Read the model definition and answer for the solid it produces. Units are mm, in the model's axes. Face numbers are marked on the shaded views. A direction names the side the tool comes from. Coordinates: 2 decimals unless noted, no trailing zeros. Order: outer loops, then holes, each group sorted by start corner. A loop starts at its lowest first (then second) coordinate and runs counter-clockwise, first axis right, second up. Notation, with made-up numbers: M 79.25,-24.75 L 115.25,-24.75 A25 ccw 115.25,11.25 Z; hole C -18.75,82.5 d5. An arc over 180 degrees is marked long. Put each result on its own line as item: value.
from build123d import *

# Parameters (mm, degrees)
SKETCH_1_W               = 15
SKETCH_1_H               = 30.8
EXTRUDE_1_DEPTH          = 1.5
SKETCH_2_W               = 15
SKETCH_2_H               = 1.5
EXTRUDE_2_DEPTH          = 9
SKETCH_3_R               = 1.25
CUT_EXTRUDE_1_DEPTH      = 1
CUT_EXTRUDE_1_DEPTH_BACK = 31.8


with BuildPart() as part:
    # 草图1 → 凸台-拉伸1 (new body)
    with BuildSketch(Plane(origin=(0, 0, 0), x_dir=(1, 0, 0), z_dir=(0, 1, 0))):
        with Locations((-5.581761006, 1.950314465)):
            Rectangle(SKETCH_1_W, SKETCH_1_H)
    extrude(amount=EXTRUDE_1_DEPTH)

    # 草图2 → 凸台-拉伸2 (add)
    with BuildSketch(Plane.XZ):
        with Locations((-5.581761006, 12.699685535)):
            Rectangle(SKETCH_2_W, SKETCH_2_H)
        with Locations((-5.581761006, -16.600314465)):
            Rectangle(SKETCH_2_W, SKETCH_2_H)
    extrude(amount=EXTRUDE_2_DEPTH)

    # 草图3 → 切除-拉伸1 (cut, two sides)
    with BuildSketch(Plane.XY.offset(13.449685535)) as cut_extrude_1_sk:
        with Locations((-9.081761006, -6)):
            Circle(SKETCH_3_R)
        with Locations((-2.081761006, -6)):
            Circle(SKETCH_3_R)
    extrude(amount=CUT_EXTRUDE_1_DEPTH, mode=Mode.SUBTRACT)
    extrude(cut_extrude_1_sk.sketch, amount=-CUT_EXTRUDE_1_DEPTH_BACK, mode=Mode.SUBTRACT)


solid = part.part
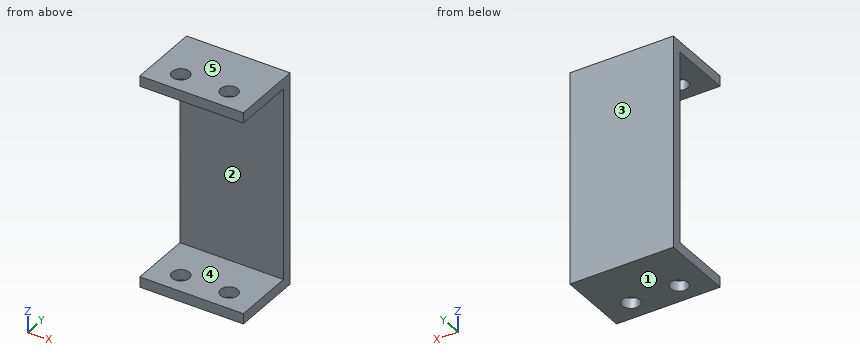
Q1. Find section A-A on y = -6. Write down the section's boundary in (x, z).
Answers below:
outline: M -13.08,-17.35 L -10.33,-17.35 L -10.33,-15.85 L -13.08,-15.85 Z; M -13.08,11.95 L -10.33,11.95 L -10.33,13.45 L -13.08,13.45 Z; M -7.83,-17.35 L -3.33,-17.35 L -3.33,-15.85 L -7.83,-15.85 Z; M -7.83,11.95 L -3.33,11.95 L -3.33,13.45 L -7.83,13.45 Z; M -0.83,-17.35 L 1.92,-17.35 L 1.92,-15.85 L -0.83,-15.85 Z; M -0.83,11.95 L 1.92,11.95 L 1.92,13.45 L -0.83,13.45 Z
Q2. Find section B-B on y = -1.25. Write down the section's boundary in (x, z), plus the area to 3 significant figures.
Answers below:
outline: M -13.08,-17.35 L 1.92,-17.35 L 1.92,-15.85 L -13.08,-15.85 Z; M -13.08,11.95 L 1.92,11.95 L 1.92,13.45 L -13.08,13.45 Z
area: 45.0 mm^2
Q3. Find section C-C on x = -9.5. Write down the section's boundary in (y, z), plus the area to 3 significant figures.
Answers below:
outline: M -9,-17.35 L -7.18,-17.35 L -7.18,-15.85 L -9,-15.85 Z; M -9,11.95 L -7.18,11.95 L -7.18,13.45 L -9,13.45 Z; M -4.82,-17.35 L 1.5,-17.35 L 1.5,13.45 L -4.82,13.45 L -4.82,11.95 L 0,11.95 L 0,-15.85 L -4.82,-15.85 Z
area: 66.1 mm^2
Q4. Find section D-D on z = 1. Write down the section's boundary in (x, y), plus the area to 3 significant figures.
Answers below:
outline: M -13.08,0 L 1.92,0 L 1.92,1.5 L -13.08,1.5 Z
area: 22.5 mm^2
Q5. Given pin 1 (2 mm diameter, centred on x = -9.08, y = -6, fed in from +Z); pin 2 (6 mm diameter, centred on x = 0, z = -9.5, fed in from -Y), each flat-ended and moving along its own axis, determine where each tip first touches the part or whether it passes through.
Answers below:
pin 1: passes through
pin 2: stops at y = 0
Q6. For a pull along Z with two mould halves and no side action, classify the marked faces 3, 4 and 5 as +Z half, -Z half, draft (parallel to the pull), parting line (faces both ways), or undercut.
Answers below:
face 3: draft
face 4: undercut
face 5: +Z half
Q7. A tool of negligible diameter and unlimited length cuts with its end or side. For the marked faces 1 and 2, from which of +Z, -Z, +X, -X, +Y, -Y can it reach the whole face along a straight path? Write none if from no direction.
Answers below:
face 1: -Z, +X, -X, +Y, -Y
face 2: +X, -X, -Y
Q8. Consider line 1 along Z through (x, y) = (-2, -8); line 2 along Y through (x, z) = (-7, -13.5). Determine where each line is inside the solid, lowest interval first.
Answers below:
line 1: z = -17.35 to -15.85, 11.95 to 13.45
line 2: y = 0 to 1.5
